For this review, take the finished solid that the model builds, in its own axes (mm). A direction names the side the tool comes from. Coordinates: 2 decimals unless noted, no trailing zeros. Loops run counter-clockwise (first coordinate to the right, second up) from the corner with the lowest first, then second, coordinate; pieces in that order, holes last. Notation, with made-up numbers: M 39,-20 L 88,-20 A25 cw 88,18 Z; hole C 15,31.5 d8. An arc over 180 degrees is marked long. Answer as a JSON object with one key per item and string values. Group by question number.
Item 1: Add section D-D (z = 0). State the section outline as (x, y) points, then the cut area to 3 significant figures.
Item 2: Add section A-A (x = 25). State the section outline as (y, z) points, then the cut area to 3 significant figures.
Item 3: Insertion check: pin 1 (10 mm diameter, centred on y = 88.5, z = 6.5, fed in from +X); pin 2 (23 mm diameter, centred on y = 94.5, z = -6.5, fed in from -X); pin 3 (6 mm diameter, centred on x = -19, y = 93.5, fed in from +Z). Each pin has a flat end and moves straight along its axis. Give the tip position at first contact, or say it passes through.
Item 4: Wall thickness on L1, parallel to Y at x = -10.5, z = -5; L2, parallel to Z at x = -1.5, y = 53; L3, parallel to X at y = 62.5, z = 18: over which ranges is each line inside the solid? List them lowest first. Write a range as from..to.
Item 5: Mouldability with a two-part tool opening along X and no side actions: class faces 6 (the face through (1, 0, 0)), 7 (the face through (0, 58, -4)), 8 (the face through (0.532, 26.989, 9.156)), 9 (the face through (-38, 11, 0)) as +X half, -X half, draft (parallel to the pull), parting line (faces both ways), or undercut.
Item 6: Add section B-B (y = 66). State the section outline as (x, z) points, then the cut area to 3 significant figures.
Item 7: Add section C-C (x = -7). State the section outline as (y, z) points, then the cut area to 3 significant figures.
Item 8: Tool access review of faces 1 (the face through (0, 58, 4)), 2 (the face through (20.757, 52.36, -13.245)), 3 (the face through (28.5, 100, 0)), 4 (the face through (24.57, 53.73, 21.06)), 5 (the face through (-28.5, 100, 0)): name each direction out of +Z, -Z, +X, -X, +Y, -Y from which nothing blocks a thin tool from reaching the whole face with its end or side.
from build123d import *

# Parameters (mm, degrees)
SKETCH1_R                = 14.25
BOSS_EXTRUDE1_DEPTH      = 28.5
BOSS_EXTRUDE2_DEPTH      = 38
BOSS_EXTRUDE3_DEPTH      = 28.5
BOSS_EXTRUDE3_DEPTH_BACK = 28.5
SKETCH3_OUTSIDE_W        = 88.718
SKETCH3_OUTSIDE_H        = 145.968
CUT_EXTRUDE1_DEPTH       = 39
BOSS_EXTRUDE5_DEPTH      = 4


with BuildPart() as part:
    # Sketch1 → Boss-Extrude1 (new body, symmetric)
    with BuildSketch(Plane(origin=(0, 0, 0), x_dir=(0, 0, -1), z_dir=(1, 0, 0))):
        with Locations((0, 100)):
            Circle(SKETCH1_R)
    extrude(amount=BOSS_EXTRUDE1_DEPTH, both=True)



with BuildPart() as body_2:
    # Sketch1<3> → Boss-Extrude2 (new body, symmetric)
    with BuildSketch(Plane(origin=(0, 0, 0), x_dir=(0, 0, -1), z_dir=(1, 0, 0))):
        with BuildLine():
            Line((-28.5, 0), (28.5, 0))
            ThreePointArc((28.5, 0), (0, 28.5), (-28.5, 0))
        make_face()
    extrude(amount=BOSS_EXTRUDE2_DEPTH, both=True)


with BuildPart() as body_3:
    # Sketch2 → Boss-Extrude3 (new body, two sides)
    with BuildSketch(Plane.XY) as boss_extrude3_sk:
        Polygon((13.444344632, 114.25), (21.5, 114.25), (35, 0), (26.944344632, 0), align=None)
    extrude(amount=BOSS_EXTRUDE3_DEPTH)
    extrude(boss_extrude3_sk.sketch, amount=-BOSS_EXTRUDE3_DEPTH_BACK)

    # Sketch3 outside → Cut-Extrude1 (cut, through all)
    with BuildSketch(Plane(origin=(0, 0, 0), x_dir=(0, 0, -1), z_dir=(1, 0, 0))):
        with Locations((0, 57.125)):
            Rectangle(SKETCH3_OUTSIDE_W, SKETCH3_OUTSIDE_H)
        Polygon((14.104575928, 102.030625), (-14.104575928, 102.030625), (-28.209151856, 4.06125), (28.209151856, 4.06125), align=None, mode=Mode.SUBTRACT)
    extrude(amount=CUT_EXTRUDE1_DEPTH, mode=Mode.SUBTRACT)


with BuildPart() as body_4:
    # Mirror1: mirrored copy
    add(body_3.part.mirror(Plane(origin=(0, 0, 0), x_dir=(0, 0, 1), z_dir=(1, 0, 0))))


with BuildPart() as part_1:
    add(part.part)

    add(body_2.part)  # Boss-Extrude5 merges body 2

    add(body_3.part)  # Boss-Extrude5 merges body 3

    add(body_4.part)  # Boss-Extrude5 merges body 4
    # Sketch4 → Boss-Extrude5 (add, symmetric)
    with BuildSketch(Plane.XY):
        Polygon((-14.888209512, 102.030625), (14.888209512, 102.030625), (26.464459512, 4.06125), (-26.464459512, 4.06125), align=None)
    extrude(amount=BOSS_EXTRUDE5_DEPTH, both=True)


solid = part_1.part
From the geometry:
{
 "1": {"outline": "M -38,0 L 38,0 L 38,28.5 L 31.63,28.5 L 24.87,85.75 L 28.5,85.75 L 28.5,114.25 L -28.5,114.25 L -28.5,85.75 L -24.87,85.75 L -31.63,28.5 L -38,28.5 Z", "area": "7,030 mm²"},
 "2": {"outline": "M 0,-28.5 A28.5 ccw 16.45,-23.27 L 16.45,-26.42 L 84.63,-16.61 L 84.63,16.61 L 16.45,26.42 L 16.45,23.27 A28.5 ccw 0,28.5 Z; C 100,0 d28.5", "area": "4,450 mm²"},
 "3": {"pin 1": "stops at x = 28.5", "pin 2": "stops at x = -28.5", "pin 3": "stops at z = 15.76"},
 "4": {"L1": "y = 0..28.06, 86.66..113.34", "L2": "z = -4..4", "L3": "x = -27.61..-19.56, 19.56..27.61"},
 "5": {"face 6": "draft", "face 7": "undercut", "face 8": "undercut", "face 9": "-X half"},
 "6": {"outline": "M -27.2,-19.29 L -19.15,-19.29 L -19.15,-4 L 19.15,-4 L 19.15,-19.29 L 27.2,-19.29 L 27.2,19.29 L 19.15,19.29 L 19.15,4 L -19.15,4 L -19.15,19.29 L -27.2,19.29 Z", "area": "928 mm²"},
 "7": {"outline": "M 0,-28.5 A28.5 ccw 28.22,-4 L 86.32,-4 A14.25 ccw long 86.32,4 L 28.22,4 A28.5 ccw 0,28.5 Z", "area": "2,370 mm²"},
 "8": {"face 1": "+Z", "face 2": "-Z", "face 3": "+Z, -Z, +X, +Y", "face 4": "+Z, +X, -X, +Y", "face 5": "+Z, -Z, -X, +Y"}
}
